Design review of the part built by this model. Coordinates are the model's own, in mm. Coordinates: 2 decimals unless noted, no trailing zeros. Use a Markdown table: item, result. Add a question column.
Q1. Wall thickness on probe 1 along Y at (x, z) = (-88.9, 4.2); probe 2 along Y at (x, z) = (62.5, 0.75); probe 3 along X at (y, z) = (54, 0.5): over which ranges is each line inside the solid? List them lowest first.
Q2. Add section A-A (x = -88.9). Count the separate pieces of the cut face and the enclosed holes in it, then the cut area to 3 significant figures.
Q3. The part is to be moulded in two halves that separate along Y. For faces 1 (the face through (-1, 72.517, 3)), 2 (the face through (-101.6, -1, 3)), 3 (the face through (62.64, 62.25, 3.13)), say which applies: pulls with the +Y half, pulls with the -Y half, needs draft (parallel to the pull), parting line crosses it, or undercut.
Q4. Insertion check: pin 1 (12.5 mm diameter, centred on x = -88.9, y = -59.817, fed in from -Z). The pin has a flat end and moves straight along its axis. Give the tip position at first contact, or say it passes through.
from build123d import *

# Parameters (mm, degrees)
SKETCH1_W                              = 203.2
SKETCH1_H                              = 145.034
BOSS_EXTRUDE1_DEPTH                    = 6.35
F_3_8_0_375_DIAMETER_HOLE1_D           = 9.525
F_3_8_0_375_DIAMETER_HOLE1_CSINK_D     = 10.795
F_3_8_0_375_DIAMETER_HOLE1_CSINK_ANGLE = 90
SKETCH4_R                              = 7
CUT_EXTRUDE1_DEPTH                     = 125.986390415


with BuildPart() as part:
    # Sketch1 → Boss-Extrude1 (new body)
    with BuildSketch(Plane.XY):
        Rectangle(SKETCH1_W, SKETCH1_H)
    extrude(amount=BOSS_EXTRUDE1_DEPTH)

    # 3/8 (0.375) Diameter Hole1 (through all)
    with Locations(Plane.XY.offset(6.35)):
        with Locations((-88.9, 59.817), (-88.9, -59.817), (88.9, -59.817), (88.9, 59.817)):
            CounterSinkHole(F_3_8_0_375_DIAMETER_HOLE1_D / 2, F_3_8_0_375_DIAMETER_HOLE1_CSINK_D / 2, counter_sink_angle=F_3_8_0_375_DIAMETER_HOLE1_CSINK_ANGLE)

    # Sketch4 → Cut-Extrude1 (cut, through all)
    with BuildSketch(Plane(origin=(0, 0, 0), x_dir=(-1, 0, 0), z_dir=(0, 0, -1))):
        with Locations((-57.483, 57.517)):
            Circle(SKETCH4_R)
        with Locations((57.517, 57.517)):
            Circle(SKETCH4_R)
        with Locations((57.517, -57.483)):
            Circle(SKETCH4_R)
        with Locations((-57.483, -57.483)):
            Circle(SKETCH4_R)
    extrude(amount=-CUT_EXTRUDE1_DEPTH, mode=Mode.SUBTRACT)


solid = part.part
Established:
| question | item | result |
|---|---|---|
| 1 | probe 1 | -72.52 to -64.58, -55.05 to 55.05, 64.58 to 72.52 |
| 1 | probe 2 | -72.52 to -62.36, -52.6 to 52.64, 62.4 to 72.52 |
| 1 | probe 3 | -101.6 to -63.57, -51.46 to 51.43, 63.54 to 101.6 |
| 2 | separate pieces | 3 |
| 2 | enclosed holes | 0 |
| 2 | area | 799 mm^2 |
| 3 | face 1 | pulls with the +Y half |
| 3 | face 2 | needs draft |
| 3 | face 3 | undercut |
| 4 | pin 1 | z = 0 |
